Can you work these out from the model? Positions are in its coordinate system, mm. A direction names the side the tool comes from. Give positions to 0.01 mm unless a question says otherwise; leave off trailing zeros. Loops run counter-clockwise (first coordinate to the right, second up) from the corner with the lowest first, then second, coordinate; pieces in that order, holes last.
from build123d import *

# Parameters (mm, degrees)
SKETCH_1_W      = 78.5
SKETCH_1_H      = 39.5
SKETCH_1_W_2    = 72.5
SKETCH_1_H_2    = 33.5
EXTRUDE_1_DEPTH = 25
SKETCH_2_W      = 108.5
SKETCH_2_H      = 69.5
EXTRUDE_2_DEPTH = 3
FILLET_1_R      = 10
CHAMFER_1_SIZE  = 6
CHAMFER_2_SIZE  = 7.5
FILLET_2_R      = 2
FILLET_3_R      = 3
FILLET_4_R      = 5
FILLET_5_R      = 1
FILLET_6_R      = 1
CHAMFER_3_SIZE  = 0.4


with BuildPart() as part:
    # 草图1 → 凸台-拉伸1 (new body)
    with BuildSketch(Plane(origin=(0, 0, 0), x_dir=(1, 0, 0), z_dir=(0, 1, 0))):
        with Locations((36.25, 16.75)):
            Rectangle(SKETCH_1_W, SKETCH_1_H)
        with Locations((36.25, 16.75)):
            Rectangle(SKETCH_1_W_2, SKETCH_1_H_2, mode=Mode.SUBTRACT)
    extrude(amount=EXTRUDE_1_DEPTH)

    # 草图2 → 凸台-拉伸2 (add)
    with BuildSketch(Plane(origin=(0, 0, 0), x_dir=(-1, 0, 0), z_dir=(0, -1, 0))):
        with Locations((-36.25, 16.75)):
            Rectangle(SKETCH_2_W, SKETCH_2_H)
    extrude(amount=EXTRUDE_2_DEPTH)

    # 圆角1
    fillet_1_edges = [part.edges().sort_by_distance(p)[0] for p in [
        (-18, -1.5, -51.5),
        (90.5, -1.5, -51.5),
        (90.5, -1.5, 18),
        (-18, -1.5, 18),
    ]]
    fillet(fillet_1_edges, radius=FILLET_1_R)

    # 倒角1
    chamfer_1_edges = [part.edges().sort_by_distance(p)[0] for p in [
        (0, 12.5, 0),
        (72.5, 12.5, 0),
    ]]
    chamfer(chamfer_1_edges, length=CHAMFER_1_SIZE)

    # 倒角2
    chamfer_2_edges = [part.edges().sort_by_distance(p)[0] for p in [
        (75.5, 12.5, 3),
        (-3, 12.5, 3),
    ]]
    chamfer(chamfer_2_edges, length=CHAMFER_2_SIZE)

    # 圆角2
    fillet_2_edges = [part.edges().sort_by_distance(p)[0] for p in [
        (0, 12.5, -33.5),
        (72.5, 12.5, -33.5),
        (6, 12.5, 0),
        (66.5, 12.5, 0),
        (72.5, 12.5, -6),
        (0, 12.5, -6),
    ]]
    fillet(fillet_2_edges, radius=FILLET_2_R)

    # 圆角3
    fillet_3_edges = [part.edges().sort_by_distance(p)[0] for p in [
        (-3, 12.5, -36.5),
        (75.5, 12.5, -36.5),
        (68, 12.5, 3),
        (4.5, 12.5, 3),
        (-3, 12.5, -4.5),
        (75.5, 12.5, -4.5),
    ]]
    fillet(fillet_3_edges, radius=FILLET_3_R)

    # 圆角4
    fillet_4_edges = [part.edges().sort_by_distance(p)[0] for p in [
        (75.5, 0, -19.621320344),
        (71.75, 0, -0.75),
        (36.25, 0, 3),
        (0.75, 0, -0.75),
        (-3, 0, -19.621320344),
        (36.25, 0, -36.5),
        (75.271638598, 0, -4.59459039),
        (67.90540961, 0, 2.771638598),
        (4.59459039, 0, 2.771638598),
        (-2.771638598, 0, -4.59459039),
        (-2.121320344, 0, -35.621320344),
        (74.621320344, 0, -35.621320344),
    ]]
    fillet(fillet_4_edges, radius=FILLET_4_R)

    # 圆角5
    fillet_5_edges = [part.edges().sort_by_distance(p)[0] for p in [
        (0, 25, -19.164213562),
        (72.5, 25, -19.164213562),
        (69.5, 25, -3),
        (3, 25, -3),
        (36.25, 25, 0),
        (0.585786438, 25, -32.914213562),
        (71.914213562, 25, -32.914213562),
        (72.347759065, 25, -6.06306026),
        (0.152240935, 25, -6.06306026),
        (6.06306026, 25, -0.152240935),
        (66.43693974, 25, -0.152240935),
        (75.5, 25, -19.621320344),
        (71.75, 25, -0.75),
        (-3, 25, -19.621320344),
        (0.75, 25, -0.75),
        (36.25, 25, 3),
        (36.25, 25, -36.5),
        (74.621320344, 25, -35.621320344),
        (-2.121320344, 25, -35.621320344),
        (-2.771638598, 25, -4.59459039),
        (4.59459039, 25, 2.771638598),
        (67.90540961, 25, 2.771638598),
        (75.271638598, 25, -4.59459039),
        (36.25, 25, -33.5),
    ]]
    fillet(fillet_5_edges, radius=FILLET_5_R)

    # 圆角6
    fillet_6_edges = [part.edges().sort_by_distance(p)[0] for p in [
        (-18, 0, -16.75),
        (36.25, 0, -51.5),
        (36.25, 0, 18),
        (90.5, 0, -16.75),
        (87.571067812, 0, 15.071067812),
        (87.571067812, 0, -48.571067812),
        (-15.071067812, 0, -48.571067812),
        (-15.071067812, 0, 15.071067812),
    ]]
    fillet(fillet_6_edges, radius=FILLET_6_R)

    # 倒角3
    chamfer_3_edges = [part.edges().sort_by_distance(p)[0] for p in [
        (-18, -3, -16.75),
        (36.25, -3, 18),
        (36.25, -3, -51.5),
        (90.5, -3, -16.75),
        (87.571067812, -3, 15.071067812),
        (87.571067812, -3, -48.571067812),
        (-15.071067812, -3, -48.571067812),
        (-15.071067812, -3, 15.071067812),
    ]]
    chamfer(chamfer_3_edges, length=CHAMFER_3_SIZE)


solid = part.part
(1) Which directions (+Z, -Z, +X, -X, +Y, -Y) give clear straight access to the entire face, cutting with the end or side of a thin tool? Please do faces 1 (the cylindrical face through (-2.14, 14.63, -35.6)), 2 (the cylindrical face through (74.6, 14.63, -35.64)), 3 (the flat face through (0.8, 14.4, -0.7)), 4 (the cylindrical face through (75.28, 14.63, -4.61)), 5 (the flat face through (36, 12, -33.5)).
Returned:
face 1: -Z, -X, +Y
face 2: -Z, +X, +Y
face 3: +Z, -X, +Y
face 4: +Z, +X, +Y
face 5: +Y
(2) Suppose I cut it at C-C on x = 51. List the corners of the cut face in (y, z) for me, plus the area to 3 significant figures.
Returned:
outline: (-3, -51.1) - (-2.6, -51.5) - (-1, -51.5) arc R1 ccw to (0, -50.5) - (0, -41.5) arc R5 cw to (5, -36.5) - (24, -36.5) arc R1 ccw to (25, -35.5) - (25, -34.5) arc R1 ccw to (24, -33.5) - (0, -33.5) - (0, 0) - (24, 0) arc R1 ccw to (25, 1) - (25, 2) arc R1 ccw to (24, 3) - (5, 3) arc R5 cw to (0, 8) - (0, 17) arc R1 ccw to (-1, 18) - (-2.6, 18) - (-3, 17.6) - close
area: 368 mm2
(3) Suppose I cut it at B-B on z = -14. List the corners of the cut face in (x, y) for me, plus the area to 3 significant figures.
Returned:
outline: (-18, -2.6) - (-17.6, -3) - (90.1, -3) - (90.5, -2.6) - (90.5, -1) arc R1 ccw to (89.5, 0) - (80.5, 0) arc R5 cw to (75.5, 5) - (75.5, 24) arc R1 ccw to (74.5, 25) - (73.5, 25) arc R1 ccw to (72.5, 24) - (72.5, 0) - (0, 0) - (0, 24) arc R1 ccw to (-1, 25) - (-2, 25) arc R1 ccw to (-3, 24) - (-3, 5) arc R5 cw to (-8, 0) - (-17, 0) arc R1 ccw to (-18, -1) - close
area: 485 mm2
(4) Will these pins go through, and if not, where does the flat tip stop? P1, Ø15, axis at x = 48.5, y = 13.5, coming from the -Z side; P2, Ø4, axis at x = 69, y = 19.5, coming from the +Z side; P3, Ø9.5, axis at y = 17, z = -26.5, coming from the +X side.
Returned:
P1: stops at z = -36.5
P2: stops at z = 2.99
P3: stops at x = 75.5
(5) Please list where these lines run through material, in increasing order: probe 1 along Z at (x, y) = (63.5, 10); probe 2 along X at (y, z) = (20, -19.5); probe 3 along Y at (x, z) = (82.5, -43).
Returned:
probe 1: z = -36.5 to -33.5, 0 to 3
probe 2: x = -3 to 0, 72.5 to 75.5
probe 3: y = -3 to 0
(6) Suppose I cut it at D-D on y = 2.5. List the corners of the cut face in (x, z) for me (3 decimals).
Returned:
outline: (-3.67, -33.5) arc R3.67 ccw to (0, -37.17) - (72.5, -37.17) arc R3.67 ccw to (76.17, -33.5) - (76.17, -5.743) arc R3.67 ccw to (75.095, -3.148) - (69.352, 2.595) arc R3.67 ccw to (66.757, 3.67) - (5.743, 3.67) arc R3.67 ccw to (3.148, 2.595) - (-2.595, -3.148) arc R3.67 ccw to (-3.67, -5.743) - close; hole (0, -31.5) arc R2 ccw to (2, -33.5) - (70.5, -33.5) arc R2 ccw to (72.5, -31.5) - (72.5, -6.828) arc R2 ccw to (71.914, -5.414) - (67.086, -0.586) arc R2 ccw to (65.672, 0) - (6.828, 0) arc R2 ccw to (5.414, -0.586) - (0.586, -5.414) arc R2 ccw to (0, -6.828) - close
(7) Suppose I cut it at A-A on y = 16.75. List the corners of the cut face in (x, z) for me.
Returned:
outline: (-3, -33.5) arc R3 ccw to (0, -36.5) - (72.5, -36.5) arc R3 ccw to (75.5, -33.5) - (75.5, -5.74) arc R3 ccw to (74.62, -3.62) - (68.88, 2.12) arc R3 ccw to (66.76, 3) - (5.74, 3) arc R3 ccw to (3.62, 2.12) - (-2.12, -3.62) arc R3 ccw to (-3, -5.74) - close; hole (0, -31.5) arc R2 ccw to (2, -33.5) - (70.5, -33.5) arc R2 ccw to (72.5, -31.5) - (72.5, -6.83) arc R2 ccw to (71.91, -5.41) - (67.09, -0.59) arc R2 ccw to (65.67, 0) - (6.83, 0) arc R2 ccw to (5.41, -0.59) - (0.59, -5.41) arc R2 ccw to (0, -6.83) - close
(8) Thinking about a two-plate mould opening in Z: for faces 6 (the flat face through (36, 14, 3)), 7 (the flat face through (37, 0, -17)), 8 (the cylindrical face through (-14.99, -1.81, -48.65)), 9 (the flat face through (0, 12, -19)), which applies, pulls with the +Z half, pulls with the -Z half, needs draft (parallel to the pull), parting line crosses it, or undercut?
Returned:
face 6: pulls with the +Z half
face 7: undercut
face 8: pulls with the -Z half
face 9: undercut
